Could you check a few things on this model? Use its own coordinates, in mm. Face numbers are marked on the shaded views. A direction names the side the tool comes from. Coordinates: 2 decimals unless noted, no trailing zeros. Loops run counter-clockwise (first coordinate to the right, second up) from the corner with the lowest first, then second, coordinate; pieces in that order, holes last. Notation, with made-up numbers: (-23.5, 13.5) -> (17.5, 13.5) arc R15 ccw to (17.5, 27.5) -> close; hole circle Ø11 at (-20, 39.5). An arc over 180 degrees is marked (long way). One line per question, with ' | ' between items.
from build123d import *

# Parameters (mm, degrees)
CYLINDER2057_R               = 1.5
CYLINDER2057_DEPTH           = 50
CYLINDER2057_PLACEMENT_ANGLE = 45
CYLINDER2056_R               = 1.5
CYLINDER2056_DEPTH           = 50
CYLINDER2056_PLACEMENT_ANGLE = 45
CYLINDER2053_R               = 1.5
CYLINDER2053_DEPTH           = 50
CYLINDER2053_PLACEMENT_ANGLE = 45
CYLINDER2055_R               = 1.5
CYLINDER2055_DEPTH           = 50
CYLINDER2055_PLACEMENT_ANGLE = 45
CYLINDER2054_R               = 3
CYLINDER2054_DEPTH           = 3
CYLINDER2054_PLACEMENT_ANGLE = 45
CYLINDER2058_R               = 3
CYLINDER2058_DEPTH           = 3
CYLINDER2058_PLACEMENT_ANGLE = 45
CYLINDER2068_R               = 3
CYLINDER2068_DEPTH           = 3
CYLINDER2068_PLACEMENT_ANGLE = 45
CYLINDER2059_R               = 3
CYLINDER2059_DEPTH           = 3
CYLINDER2059_PLACEMENT_ANGLE = 45
CYLINDER2048_R               = 8
CYLINDER2048_DEPTH           = 6
CYLINDER2045_R               = 3
CYLINDER2045_DEPTH           = 50
CYLINDER2060_R               = 3
CYLINDER2060_DEPTH           = 50
CYLINDER2046_R               = 1.5
CYLINDER2046_DEPTH           = 50
CYLINDER2044_R               = 1.5
CYLINDER2044_DEPTH           = 50
CYLINDER2042_R               = 74
CYLINDER2042_DEPTH           = 15
CYLINDER2047_R               = 46
CYLINDER2047_DEPTH           = 36
CYLINDER2043_R               = 46
CYLINDER2043_DEPTH           = 36
BOX988_W                     = 148
BOX988_H                     = 38
BOX988_DEPTH                 = 15
CHAMFER078_SIZE              = 2


with BuildPart() as obj1:
    # Cylinder2057 → Cylinder2057 (new body)
    with BuildSketch(Plane.XY):
        Circle(CYLINDER2057_R)
    extrude(amount=CYLINDER2057_DEPTH)


with BuildPart() as obj1_1:
    # Cylinder2057 placement: moved
    add(obj1.part.moved(Location((-31, 77, 0))).rotate(Axis((-31, 77, 0), (0, 0, 1)), CYLINDER2057_PLACEMENT_ANGLE))


with BuildPart() as compound960:
    # Cylinder2056 → Cylinder2056 (new body)
    with BuildSketch(Plane.XY):
        Circle(CYLINDER2056_R)
    extrude(amount=CYLINDER2056_DEPTH)


with BuildPart() as compound960_1:
    # Cylinder2056 placement: moved
    add(compound960.part.moved(Location((31, 77, 0))).rotate(Axis((31, 77, 0), (0, 0, 1)), CYLINDER2056_PLACEMENT_ANGLE))

    # Compound960: union obj1
    add(obj1_1.part)


with BuildPart() as obj2:
    # Cylinder2053 → Cylinder2053 (new body)
    with BuildSketch(Plane.XY):
        Circle(CYLINDER2053_R)
    extrude(amount=CYLINDER2053_DEPTH)


with BuildPart() as obj2_1:
    # Cylinder2053 placement: moved
    add(obj2.part.moved(Location((-54, 59, 0))).rotate(Axis((-54, 59, 0), (0, 0, 1)), CYLINDER2053_PLACEMENT_ANGLE))


with BuildPart() as compound1089:
    # Cylinder2055 → Cylinder2055 (new body)
    with BuildSketch(Plane.XY):
        Circle(CYLINDER2055_R)
    extrude(amount=CYLINDER2055_DEPTH)


with BuildPart() as compound1089_1:
    # Cylinder2055 placement: moved
    add(compound1089.part.moved(Location((54, 59, 0))).rotate(Axis((54, 59, 0), (0, 0, 1)), CYLINDER2055_PLACEMENT_ANGLE))

    # Compound959: union obj2
    add(obj2_1.part)

    # Compound1089: union Compound960
    add(compound960_1.part)


with BuildPart() as obj3:
    # Cylinder2054 → Cylinder2054 (new body)
    with BuildSketch(Plane.XY):
        Circle(CYLINDER2054_R)
    extrude(amount=CYLINDER2054_DEPTH)


with BuildPart() as obj3_1:
    # Cylinder2054 placement: moved
    add(obj3.part.moved(Location((-31, 77, 0))).rotate(Axis((-31, 77, 0), (0, 0, 1)), CYLINDER2054_PLACEMENT_ANGLE))


with BuildPart() as compound1105:
    # Cylinder2058 → Cylinder2058 (new body)
    with BuildSketch(Plane.XY):
        Circle(CYLINDER2058_R)
    extrude(amount=CYLINDER2058_DEPTH)


with BuildPart() as compound1105_1:
    # Cylinder2058 placement: moved
    add(compound1105.part.moved(Location((31, 77, 0))).rotate(Axis((31, 77, 0), (0, 0, 1)), CYLINDER2058_PLACEMENT_ANGLE))

    # Compound1105: union obj3
    add(obj3_1.part)


with BuildPart() as obj4:
    # Cylinder2068 → Cylinder2068 (new body)
    with BuildSketch(Plane.XY):
        Circle(CYLINDER2068_R)
    extrude(amount=CYLINDER2068_DEPTH)


with BuildPart() as obj4_1:
    # Cylinder2068 placement: moved
    add(obj4.part.moved(Location((-54, 59, 0))).rotate(Axis((-54, 59, 0), (0, 0, 1)), CYLINDER2068_PLACEMENT_ANGLE))


with BuildPart() as compound1098:
    # Cylinder2059 → Cylinder2059 (new body)
    with BuildSketch(Plane.XY):
        Circle(CYLINDER2059_R)
    extrude(amount=CYLINDER2059_DEPTH)


with BuildPart() as compound1098_1:
    # Cylinder2059 placement: moved
    add(compound1098.part.moved(Location((54, 59, 0))).rotate(Axis((54, 59, 0), (0, 0, 1)), CYLINDER2059_PLACEMENT_ANGLE))

    # Compound965: union obj4
    add(obj4_1.part)

    # Compound1098: union Compound1105
    add(compound1105_1.part)


with BuildPart() as compound1098_2:
    # Compound1098 placement: moved
    add(compound1098_1.part.moved(Location((0, 0, 16))))


with BuildPart() as obj5:
    # Cylinder2048 → Cylinder2048 (new body)
    with BuildSketch(Plane(origin=(0, 83, 25), x_dir=(1, 0, 0), z_dir=(0, 0, 1))):
        Circle(CYLINDER2048_R)
    extrude(amount=CYLINDER2048_DEPTH)


with BuildPart() as obj6:
    # Cylinder2045 → Cylinder2045 (new body)
    with BuildSketch(Plane(origin=(-71, 106, 24), x_dir=(1, 0, 0), z_dir=(0, -1, 0))):
        Circle(CYLINDER2045_R)
    extrude(amount=CYLINDER2045_DEPTH)


with BuildPart() as compound955:
    # Cylinder2060 → Cylinder2060 (new body)
    with BuildSketch(Plane(origin=(71, 106, 24), x_dir=(1, 0, 0), z_dir=(0, -1, 0))):
        Circle(CYLINDER2060_R)
    extrude(amount=CYLINDER2060_DEPTH)

    # Compound955: union obj6
    add(obj6.part)


with BuildPart() as obj7:
    # Cylinder2046 → Cylinder2046 (new body)
    with BuildSketch(Plane(origin=(-71, 80, 24), x_dir=(1, 0, 0), z_dir=(0, -1, 0))):
        Circle(CYLINDER2046_R)
    extrude(amount=CYLINDER2046_DEPTH)


with BuildPart() as compound953:
    # Cylinder2044 → Cylinder2044 (new body)
    with BuildSketch(Plane(origin=(71, 80, 24), x_dir=(1, 0, 0), z_dir=(0, -1, 0))):
        Circle(CYLINDER2044_R)
    extrude(amount=CYLINDER2044_DEPTH)

    # Compound953: union obj7
    add(obj7.part)


with BuildPart() as obj8:
    # Cylinder2042 → Cylinder2042 (new body)
    with BuildSketch(Plane.XY.offset(16)):
        Circle(CYLINDER2042_R)
    extrude(amount=CYLINDER2042_DEPTH)


with BuildPart() as obj9:
    # Cylinder2047 → Cylinder2047 (new body)
    with BuildSketch(Plane(origin=(76.3, 104, 16), x_dir=(1, 0, 0), z_dir=(0, 0, 1))):
        Circle(CYLINDER2047_R)
    extrude(amount=CYLINDER2047_DEPTH)


with BuildPart() as obj10:
    # Cylinder2043 → Cylinder2043 (new body)
    with BuildSketch(Plane(origin=(-76.3, 104, 16), x_dir=(1, 0, 0), z_dir=(0, 0, 1))):
        Circle(CYLINDER2043_R)
    extrude(amount=CYLINDER2043_DEPTH)


with BuildPart() as cut686:
    # Box988 → Box988 (new body)
    with BuildSketch(Plane(origin=(-74, 48, 16), x_dir=(1, 0, 0), z_dir=(0, 0, 1))):
        with Locations((74, 19)):
            Rectangle(BOX988_W, BOX988_H)
    extrude(amount=BOX988_DEPTH)

    # Cut701: cut obj10
    add(obj10.part, mode=Mode.SUBTRACT)

    # Cut695: cut obj9
    add(obj9.part, mode=Mode.SUBTRACT)

    # Cut699: cut obj8
    add(obj8.part, mode=Mode.SUBTRACT)

    # Cut685: cut Compound953
    add(compound953.part, mode=Mode.SUBTRACT)

    # Cut697: cut Compound955
    add(compound955.part, mode=Mode.SUBTRACT)

    # Cut687: cut obj5
    add(obj5.part, mode=Mode.SUBTRACT)

    # Chamfer078
    chamfer078_edges = [cut686.edges().sort_by_distance(p)[0] for p in [
        (0, 86, 16),
    ]]
    chamfer(chamfer078_edges, length=CHAMFER078_SIZE)

    # Cut689: cut Compound1098
    add(compound1098_2.part, mode=Mode.SUBTRACT)

    # Cut686: cut Compound1089
    add(compound1089_1.part, mode=Mode.SUBTRACT)


solid = cut686.part
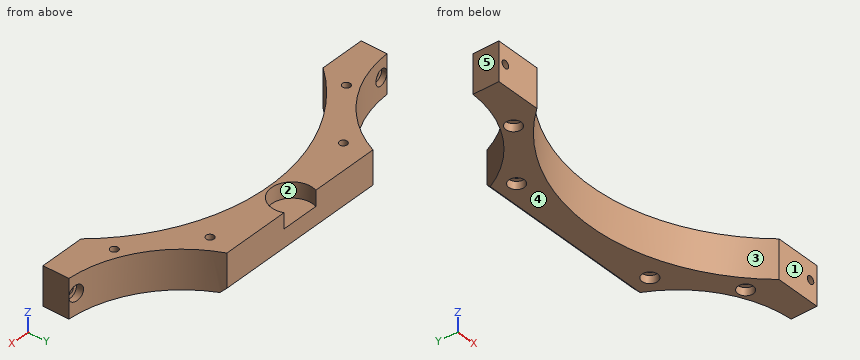
1) I need wall thicknesses on line 1 along Z through (x, y) = (-71, 52); line 2 along Z through (x, y) = (71, 57.8); line 3 along X through (y, z) = (55, 23.25). Which ranges of each line are inside material? Lowest first, please. Write a range as from..to.
Data:
line 1: 16..22.5, 25.5..31 | line 2: 16..21, 27..31 | line 3: -74..-72.3, -69.7..-49.51, 49.51..69.7, 72.3..74
2) If we section it at A-A on x = 0: Please give me the cut outline in (y, z), and give its area (3 significant figures).
Data:
outline: (74, 16) -> (84, 16) -> (86, 18) -> (86, 25) -> (75, 25) -> (75, 31) -> (74, 31) -> close | area: 112 mm²
3) If we section it at C-C on y = 52: Please give me the cut outline in (x, z), and give its area (3 significant figures).
Data:
outline: (-74, 16) -> (-52.65, 16) -> (-52.65, 31) -> (-74, 31) -> close; (52.65, 16) -> (74, 16) -> (74, 31) -> (52.65, 31) -> close; hole circle Ø3 at (-71, 24); hole circle Ø3 at (71, 24) | area: 626 mm²
4) If we section it at D-D on x = -71: Please give me the cut outline in (y, z), and give its area (3 significant figures).
Data:
outline: (48, 16) -> (58.31, 16) -> (58.31, 21) -> (56, 21) -> (56, 22.5) -> (48, 22.5) -> close; (48, 25.5) -> (56, 25.5) -> (56, 27) -> (58.31, 27) -> (58.31, 31) -> (48, 31) -> close | area: 117 mm²
5) We'd pull the mould along X, two halves only. Please class the marked faces 3, 4 and 5: pulls with the +X half, pulls with the -X half, needs draft (parallel to the pull), parting line crosses it, or undercut.
Data:
face 3: undercut | face 4: needs draft | face 5: pulls with the -X half
6) I'm going to push flat-ended pins straight in: pin 1 Ø1.8 at (x, z) = (70, 24.5) entering from +Y; pin 2 Ø5 at (x, z) = (-72, 25.5) entering from +Y (3 decimals); pin 3 Ø6 at (y, z) = (66, 25.5) entering from +X. Where does each tip first touch, or does it pass through?
Data:
pin 1: y = 56 | pin 2: y = 58.455 | pin 3: x = 55.44
7) If we section it at B-B on y = 67.5: Please give me the cut outline in (x, z), and give its area (3 significant figures).
Data:
outline: (-48.3, 16) -> (-30.33, 16) -> (-30.33, 31) -> (-48.3, 31) -> close; (30.33, 16) -> (48.3, 16) -> (48.3, 31) -> (30.33, 31) -> close | area: 539 mm²
8) On a 3-axis mill with a long thin cutter (end or side, diameter ignored), from which of +Z, -Z, +X, -X, +Y, -Y can I reach the whole of each face in a straight line? I mean the marked faces 1 and 2. Say none if no direction works.
Data:
face 1: +Z, -Z, +X, -X, -Y | face 2: +Z
